from build123d import *

# Parameters (mm, degrees)
BOSS_EXTRUDE2_DEPTH  = 2.5
BOSS_EXTRUDE3_START  = 5
BOSS_EXTRUDE3_DEPTH  = 5
M3_CLEARANCE_HOLE1_D = 3.6


with BuildPart() as part:
    # Sketch2 → Boss-Extrude2 (new body)
    # profile 1 of 2: a face of its own
    with BuildSketch(Plane.XY.offset(-2000)):
        with BuildLine():
            Line((102.89897186, 166.585877116), (133.89897186, 166.585877116))
            ThreePointArc((133.89897186, 166.585877116), (139.202272719, 164.389177975), (141.39897186, 159.085877116))
            Line((141.39897186, 159.085877116), (141.39897186, 138.785877116))
            Line((141.39897186, 138.785877116), (141.39897186, 135.685877116))
            Line((141.39897186, 135.685877116), (141.39897186, 135.385877116))
            Line((141.39897186, 135.385877116), (141.39897186, 133.385877116))
            Line((141.39897186, 133.385877116), (141.39897186, 133.085877116))
            Line((141.39897186, 133.085877116), (141.39897186, 131.333076667))
            Line((141.39897186, 131.333076667), (141.39897186, 128.085877116))
            ThreePointArc((141.39897186, 128.085877116), (139.202272719, 122.782576257), (133.89897186, 120.585877116))
            Line((133.89897186, 120.585877116), (102.89897186, 120.585877116))
            ThreePointArc((102.89897186, 120.585877116), (97.595671001, 122.782576257), (95.39897186, 128.085877116))
            Line((95.39897186, 128.085877116), (95.39897186, 159.085877116))
            ThreePointArc((95.39897186, 159.085877116), (97.595671001, 164.389177975), (102.89897186, 166.585877116))
        make_face()
        with BuildLine():
            ThreePointArc((138.89897186, 159.085877116), (137.434505766, 162.621411022), (133.89897186, 164.085877116))
            Line((133.89897186, 164.085877116), (102.89897186, 164.085877116))
            ThreePointArc((102.89897186, 164.085877116), (99.363437954, 162.621411022), (97.89897186, 159.085877116))
            Line((97.89897186, 159.085877116), (97.89897186, 128.085877116))
            ThreePointArc((97.89897186, 128.085877116), (99.363437954, 124.55034321), (102.89897186, 123.085877116))
            Line((102.89897186, 123.085877116), (133.89897186, 123.085877116))
            ThreePointArc((133.89897186, 123.085877116), (137.434505766, 124.55034321), (138.89897186, 128.085877116))
            Line((138.89897186, 128.085877116), (138.89897186, 131.333076667))
            Line((138.89897186, 131.333076667), (138.89897186, 133.085877116))
            Line((138.89897186, 133.085877116), (138.89897186, 133.385877116))
            Line((138.89897186, 133.385877116), (138.89897186, 135.385877116))
            Line((138.89897186, 135.385877116), (138.89897186, 135.685877116))
            Line((138.89897186, 135.685877116), (138.89897186, 138.785877116))
            Line((138.89897186, 138.785877116), (138.89897186, 159.085877116))
        make_face(mode=Mode.SUBTRACT)
    # profile 2 of 2: a face of its own
    with BuildSketch(Plane.XY.offset(-2000)):
        with BuildLine():
            Line((138.89897186, 135.685877116), (138.89897186, 138.785877116))
            Line((138.89897186, 138.785877116), (138.89897186, 159.085877116))
            ThreePointArc((138.89897186, 159.085877116), (137.434505766, 162.621411022), (133.89897186, 164.085877116))
            Line((133.89897186, 164.085877116), (102.89897186, 164.085877116))
            ThreePointArc((102.89897186, 164.085877116), (99.363437954, 162.621411022), (97.89897186, 159.085877116))
            Line((97.89897186, 159.085877116), (97.89897186, 128.085877116))
            ThreePointArc((97.89897186, 128.085877116), (99.363437954, 124.55034321), (102.89897186, 123.085877116))
            Line((102.89897186, 123.085877116), (133.89897186, 123.085877116))
            ThreePointArc((133.89897186, 123.085877116), (137.434505766, 124.55034321), (138.89897186, 128.085877116))
            Line((138.89897186, 128.085877116), (138.89897186, 131.333076667))
            Line((138.89897186, 131.333076667), (138.89897186, 133.085877116))
            Line((138.89897186, 133.085877116), (138.89897186, 133.385877116))
            Line((138.89897186, 133.385877116), (138.89897186, 135.385877116))
            Line((138.89897186, 135.385877116), (138.89897186, 135.685877116))
        make_face()
        with BuildLine():
            ThreePointArc((99.460267487, 142.060925747), (99.432576344, 142.456345732), (99.413140247, 142.85225734))
            ThreePointArc((99.413140247, 142.85225734), (99.62769877, 146.525146856), (100.54610998, 150.087824725))
            ThreePointArc((100.54610998, 150.087824725), (102.540191704, 154.050058497), (105.398627834, 157.441960805))
            ThreePointArc((105.398627834, 157.441960805), (125.948589847, 161.021566614), (137.39897186, 143.585877116))
            ThreePointArc((137.39897186, 143.585877116), (123.543114722, 125.295502757), (102.184467206, 133.681845673))
            ThreePointArc((102.184467206, 133.681845673), (100.329957721, 137.711293892), (99.460267487, 142.060925747))
        make_face(mode=Mode.SUBTRACT)
    extrude(amount=BOSS_EXTRUDE2_DEPTH)

    # Sketch4 → Boss-Extrude3 (add)
    with BuildSketch(Plane(origin=(0, 0, -2000), x_dir=(-1, 0, 0), z_dir=(0, 0, -1)).offset(BOSS_EXTRUDE3_START)):
        with BuildLine():
            Line((-102.89897186, 166.585877116), (-133.89897186, 166.585877116))
            ThreePointArc((-133.89897186, 166.585877116), (-139.202272719, 164.389177975), (-141.39897186, 159.085877116))
            Line((-141.39897186, 159.085877116), (-141.39897186, 128.085877116))
            ThreePointArc((-141.39897186, 128.085877116), (-139.202272719, 122.782576257), (-133.89897186, 120.585877116))
            Line((-133.89897186, 120.585877116), (-102.89897186, 120.585877116))
            ThreePointArc((-102.89897186, 120.585877116), (-97.595671001, 122.782576257), (-95.39897186, 128.085877116))
            Line((-95.39897186, 128.085877116), (-95.39897186, 159.085877116))
            ThreePointArc((-95.39897186, 159.085877116), (-97.595671001, 164.389177975), (-102.89897186, 166.585877116))
        make_face()
        with BuildLine():
            Line((-102.89897186, 164.085877116), (-133.89897186, 164.085877116))
            ThreePointArc((-133.89897186, 164.085877116), (-137.434505766, 162.621411022), (-138.89897186, 159.085877116))
            Line((-138.89897186, 159.085877116), (-138.89897186, 128.085877116))
            ThreePointArc((-138.89897186, 128.085877116), (-137.434505766, 124.55034321), (-133.89897186, 123.085877116))
            Line((-133.89897186, 123.085877116), (-102.89897186, 123.085877116))
            ThreePointArc((-102.89897186, 123.085877116), (-99.363437954, 124.55034321), (-97.89897186, 128.085877116))
            Line((-97.89897186, 128.085877116), (-97.89897186, 159.085877116))
            ThreePointArc((-97.89897186, 159.085877116), (-99.363437954, 162.621411022), (-102.89897186, 164.085877116))
        make_face(mode=Mode.SUBTRACT)
    extrude(amount=-BOSS_EXTRUDE3_DEPTH)

    # M3 Clearance Hole1 (through all)
    with Locations(Plane.XY.offset(-1997.5)):
        with Locations((102.39897186, 159.585877116), (102.39897186, 127.585877116), (134.39897186, 127.585877116), (134.39897186, 159.585877116)):
            Hole(M3_CLEARANCE_HOLE1_D / 2)


solid = part.part
The model under review builds one solid part; all positions refer to its coordinate system, in mm. A direction names the side the tool comes from. Round coordinates to 2 decimals unless told otherwise and drop trailing zeros. Loops run counter-clockwise (first coordinate to the right, second up) from the corner with the lowest first, then second, coordinate; pieces in that order, holes last. Notation, with made-up numbers: (10.25, 19.25) -> (61.25, 19.25) arc R4 cw to (61.25, 25.25) -> close; hole circle Ø11 at (87.5, -18.75). An arc over 180 degrees is marked (long way). Return JSON: item names as keys, results as strings.
(1) For faces 4 (the cylindrical face through (101.431, 161.104, -1998.768)), 5 (the cylindrical face through (99.32, 162.58, -2002.54)), list the 3-axis set-ups (+Z, -Z, +X, -X, +Y, -Y) from which the entire face can be reached by the end or side of a thin tool; tool diameter is ignored.
Solved:
{"face 4": "+Z, -Z", "face 5": "-Z"}
(2) The part is to be moulded in two halves that separate along Y. For faces 1 (the cylindrical face through (99.403, 124.512, -2002.535)), 2 (the flat face through (141.399, 144, -2001)), 3 (the cylindrical face through (97.654, 122.725, -2001.302)), say which applies: released by +Y, released by -Y, zero draft, split by the parting line, or undercut.
Solved:
{"face 1": "undercut", "face 2": "zero draft", "face 3": "released by -Y"}
(3) For line 1 (X direction, y = 129, z = -2003.5); line 2 (Y direction, x = 110, z = -2000.25); line 3 (Y direction, x = 103.5, z = -1998), list the stretches that pass through material, from the lowest coordinate up.
Solved:
{"line 1": "95.4 to 97.9, 138.9 to 141.4", "line 2": "120.59 to 123.09, 164.09 to 166.59", "line 3": "120.59 to 126.16, 129.01 to 131.8, 155.38 to 158.16, 161.01 to 166.59"}
(4) Add section B-B on x = 127.5. Write out the cut boundary in (y, z).
Solved:
{"outline": "(120.59, -2005) -> (123.09, -2005) -> (123.09, -2000) -> (126.91, -2000) -> (126.91, -1997.5) -> (120.59, -1997.5) -> close; (160.26, -2000) -> (164.09, -2000) -> (164.09, -2005) -> (166.59, -2005) -> (166.59, -1997.5) -> (160.26, -1997.5) -> close"}
(5) Add section C-C on y = 154. Write out the cut boundary in (x, z).
Solved:
{"outline": "(95.4, -2005) -> (97.9, -2005) -> (97.9, -2000) -> (102.51, -2000) -> (102.51, -1997.5) -> (95.4, -1997.5) -> close; (134.29, -2000) -> (138.9, -2000) -> (138.9, -2005) -> (141.4, -2005) -> (141.4, -1997.5) -> (134.29, -1997.5) -> close"}
(6) For pin 1 (3 mm diameter, centred on x = 102.4, y = 127.59, fed in from -Z); pin 2 (1 mm diameter, centred on x = 136.5, y = 154, fed in from -Z), all flat-tipped, find the tip position at first contact; note any pin that passes through.
Solved:
{"pin 1": "through", "pin 2": "z = -2000"}
(7) Add section D-D on x = 135.5. Write out the cut boundary in (y, z).
Solved:
{"outline": "(120.76, -2005) -> (123.35, -2005) -> (123.35, -2000) -> (126.16, -2000) -> (126.16, -1997.5) -> (120.76, -1997.5) -> close; (129.01, -2000) -> (135.31, -2000) -> (135.31, -1997.5) -> (129.01, -1997.5) -> close; (151.87, -2000) -> (158.16, -2000) -> (158.16, -1997.5) -> (151.87, -1997.5) -> close; (161.01, -2000) -> (163.82, -2000) -> (163.82, -2005) -> (166.41, -2005) -> (166.41, -1997.5) -> (161.01, -1997.5) -> close"}
(8) Add section A-A on z = -2001.5. Write out the cut boundary in (x, y).
Solved:
{"outline": "(95.4, 128.09) arc R7.5 ccw to (102.9, 120.59) -> (133.9, 120.59) arc R7.5 ccw to (141.4, 128.09) -> (141.4, 159.09) arc R7.5 ccw to (133.9, 166.59) -> (102.9, 166.59) arc R7.5 ccw to (95.4, 159.09) -> close; hole (97.9, 128.09) arc R5 ccw to (102.9, 123.09) -> (133.9, 123.09) arc R5 ccw to (138.9, 128.09) -> (138.9, 159.09) arc R5 ccw to (133.9, 164.09) -> (102.9, 164.09) arc R5 ccw to (97.9, 159.09) -> close"}
